from build123d import *

# Parameters (mm, degrees)
SKETCH1_R      = 19.5
SKETCH1_R_2    = 18
EXTRUDE1_DEPTH = 139.7
EXTRUDE2_START = 19.9898
SKETCH2_R      = 62.446297133
SKETCH2_R_2    = 18
EXTRUDE2_DEPTH = 19.9898


with BuildPart() as part:
    # Sketch1 → Extrude1 (new body)
    with BuildSketch(Plane.XY):
        Circle(SKETCH1_R)
        Circle(SKETCH1_R_2, mode=Mode.SUBTRACT)
    extrude(amount=-EXTRUDE1_DEPTH)

    # Sketch2 → Extrude2 (add)
    with BuildSketch(Plane.XY.offset(EXTRUDE2_START)):
        Circle(SKETCH2_R)
        Circle(SKETCH2_R_2, mode=Mode.SUBTRACT)
    extrude(amount=-EXTRUDE2_DEPTH)

    # Sketch3 → Revolve1 (revolve)
    with BuildSketch(Plane(origin=(0, 0, 0), x_dir=(0, 0, -1), z_dir=(1, 0, 0)), mode=Mode.PRIVATE) as revolve1_sk:
        Polygon((139.7, 18), (139.7, 14.5), (136.2, 18), align=None)
    revolve(revolve1_sk.sketch.rotate(Axis((0, 0, -143.10013627), (0, 0, 1)), 270), axis=Axis((0, 0, -143.10013627), (0, 0, 1)))


solid = part.part
Verification items for the finished model (mm, model axes). A direction names the side the tool comes from. Give positions to 0.01 mm unless a question says otherwise; leave off trailing zeros. Write each loop counter-clockwise with the first axis right and the second up, starting at its lowest first coordinate (ties: lowest second). Pieces come first, ordered by that corner, then holes. Notation, with made-up numbers: M -15.5,5.5 L -6.5,5.5 A24 cw -6.5,21.5 Z; hole C 53.25,73 d5. An arc over 180 degrees is marked long. Put each result on its own line as item: value. Start each with the question number.
1. Go/stop test with flat-tipped pins: pin 1 Ø5 at (x, y) = (16, 49.5) entering from -Z; pin 2 Ø3 at (x, z) = (-9, -38.5) entering from +Y; pin 3 Ø1 at (x, z) = (12.5, -80.5) entering from +Y. Record where each tip stops, or that it passes through.
2. Set-up check for faces 5 (the face through (0, 15, -139.7)), 6 (the face through (-15, -13, 0)): record each of +Z, -Z, +X, -X, +Y, -Y from which the full face is reachable in a straight line by a thin tool's end or side.
3. Section check D-D (x = 35). Record the cut outline in (y, z).
4. Section check C-C (z = -114.5). Record the cut outline in (x, y).
5. Section check A-A (y = 0). Record the cut outline in (x, z).
6. Scan lines: line 1 along Y through (x, z) = (0, -18); line 2 along Z through (x, y) = (-18, -44.5); line 3 along X through (y, z) = (7, 6). Record each from-to range of solid material in increasing order. Write a range as [from, to].
7. Draft check along Y on faces 1 (the face through (-1.916, 14.594, -139.481)), 2 (the face through (-13.54, -60.96, 10.13)), 3 (the face through (-2.343, 17.847, -57.012)), 4 (the face through (13, -13, 19.99)). Enter one of: +Y half, -Y half, draft (parallel to the pull), parting line (faces both ways), or undercut.
Answer list:
1. pin 1: z = 0
1. pin 2: y = 18
1. pin 3: y = 15.37
2. face 5: -Z, +X, -X, +Y, -Y
2. face 6: -Z
3. outline: M -51.72,0 L 51.72,0 L 51.72,19.99 L -51.72,19.99 Z
4. outline: C 0,0 d39; hole C 0,0 d36
5. outline: M -62.45,0 L -19.5,0 L -19.5,-139.7 L -14.5,-139.7 L -18,-136.2 L -18,19.99 L -62.45,19.99 Z; M 14.5,-139.7 L 19.5,-139.7 L 19.5,0 L 62.45,0 L 62.45,19.99 L 18,19.99 L 18,-136.2 Z
6. line 1: [-19.5, -18], [18, 19.5]
6. line 2: [0, 19.99]
6. line 3: [-62.05, -16.58], [16.58, 62.05]
7. face 1: undercut
7. face 2: parting line
7. face 3: undercut
7. face 4: draft
